Verification items for the finished model (mm, model axes). A direction names the side the tool comes from. Give positions to 0.01 mm unless a question says otherwise; leave off trailing zeros. Write each loop counter-clockwise with the first axis right and the second up, starting at its lowest first coordinate (ties: lowest second). Pieces come first, ordered by that corner, then holes. Notation, with made-up numbers: M 73,8.25 L 123,8.25 A6 cw 123,19.25 Z; hole C 74.25,18 d4. An arc over 180 degrees is marked long. Write item = value, one per line.
from build123d import *

# Parameters (mm, degrees)
F0_R     = 22.5
F0_R_2   = 3
F1_DEPTH = 59
F2_DEPTH = 93.8
F3_R     = 1.5
F4_DEPTH = 3


with BuildPart() as f1:
    # F0 (on Front) → F1 (new body)
    with BuildSketch(Plane.XZ):
        with Locations((-27.658976, 18.853478)):
            Circle(F0_R)
        with Locations((-27.658976, 18.853478)):
            Circle(F0_R_2, mode=Mode.SUBTRACT)
    extrude(amount=F1_DEPTH)

    # F0 (on Front) → F2 (join)
    with BuildSketch(Plane.XZ):
        with Locations((-27.658976, 18.853478)):
            Circle(F0_R_2)
    extrude(amount=F2_DEPTH)

    # F3 (on face) → F4 (cut)
    with BuildSketch(Plane.XZ.offset(59)):
        with Locations((-27.658976, 31.353478)):
            Circle(F3_R)
        with Locations((-40.158976, 18.853478)):
            Circle(F3_R)
        with Locations((-27.658976, 6.353478)):
            Circle(F3_R)
        with Locations((-15.158976, 18.853478)):
            Circle(F3_R)
    extrude(amount=-F4_DEPTH, mode=Mode.SUBTRACT)


solid = f1.part
1) Material ranges on probe 1 along Y at (x, z) = (-39, 4.5); probe 2 along X at (y, z) = (-53.5, 29); probe 3 along Z at (x, y) = (-38.5, -35), recorded low to high. Write a range as from..to.
From the geometry:
probe_1 = -59..0
probe_2 = -47.74..-7.58
probe_3 = -0.86..38.57
2) Tool access check on faces 4 (the cylindrical face through (-41.26, -57.52, 19.87)), 5 (the flat face through (-28, 0, 19)). Record the directions out of +Z, -Z, +X, -X, +Y, -Y that give a thin tool (end or side, any length) a straight path to the whole face; none if there is none.
From the geometry:
face_4 = -Y
face_5 = +Z, -Z, +X, -X, +Y
3) Cross-section at C-C on y = -52. Record the boundary of the cut face in (x, z).
From the geometry:
outline = C -27.66,18.85 d45
4) Depth check by flat-ended pin: P1, Ø4, axis at x = -26, y = -28, coming from the -Z side; P2, Ø2.5, axis at x = -40.5, z = 19, coming from the -Y side; P3, Ø2.5, axis at x = -15.16, z = 18.85, coming from the +Y side; P4, Ø6, axis at x = -10, y = -50, coming from the +Z side. Enter the tip coordinate at first touch or a pass-through.
From the geometry:
P1 = -3.65
P2 = -59
P3 = 0
P4 = 35.92
5) Cross-section at D-D on x = -22. Record the boundary of the cut face in (y, z).
From the geometry:
outline = M -59,-2.92 L 0,-2.92 L 0,40.63 L -59,40.63 Z
6) Cross-section at A-A on x = -28. Record the boundary of the cut face in (y, z).
From the geometry:
outline = M -93.8,15.87 L -59,15.87 L -59,7.81 L -56,7.81 L -56,4.89 L -59,4.89 L -59,-3.64 L 0,-3.64 L 0,41.35 L -59,41.35 L -59,32.81 L -56,32.81 L -56,29.89 L -59,29.89 L -59,21.83 L -93.8,21.83 Z
7) Draft check along Z on faces 1 (the cylindrical face through (-6.198, -29.087, 25.612)), 2 (the flat face through (-28, -56, 31)), 3 (the flat face through (-23, -59, 19)). Enter one of: +Z half, -Z half, draft (parallel to the pull), parting line (faces both ways), or undercut.
From the geometry:
face_1 = parting line
face_2 = undercut
face_3 = draft
8) Cross-section at B-B on z = 38. Record the boundary of the cut face in (x, y), plus the area to 3 significant figures.
From the geometry:
outline = M -39.48,-59 L -15.84,-59 L -15.84,0 L -39.48,0 Z
area = 1,390 mm^2
